from build123d import *

# Parameters (mm, degrees)
F0_W     = 73.131912
F0_H     = 3.448933
F1_DEPTH = 19.05


with BuildPart() as f1:
    # F0 (on Front) → F1 (new body)
    with BuildSketch(Plane.XZ):
        with Locations((-0.653278, -1.724466)):
            Rectangle(F0_W, F0_H)
        Polygon((-37.219234, 0), (-38.690276, 0), (-38.690276, -56.196377), (-37.219234, -56.196377), (-37.219234, -3.448933), align=None)
    extrude(amount=F1_DEPTH)


solid = f1.part
Work out the finished part from the listing and answer in its coordinate system (mm). A direction names the side the tool comes from. Coordinates: 2 decimals unless noted, no trailing zeros. Order: outer loops, then holes, each group sorted by start corner. A loop starts at its lowest first (then second) coordinate and runs counter-clockwise, first axis right, second up. Notation, with made-up numbers: (78.25, 55) - (122.25, 55) arc R19 ccw to (122.25, 84) - close; hole circle Ø5 at (-29.75, 7). An arc over 180 degrees is marked (long way). Put each result on its own line as item: value. Start each with the question number.
1) Find the intervals of material crossed by line 1 (Z direction, x = 23, y = -13.75); line 2 (X direction, y = -12, z = -33), in increasing order. Write a range as from..to.
2) Find section C-C (x = -31). Give the vertices of the cut face in (y, z).
3) Flat-ended cylindrical pins translate along their axes: pin 1 (1 mm diameter, centred on x = 24.5, y = -14, fed in from -Z); pin 2 (1.5 mm diameter, centred on y = -5.5, z = -40.5, fed in from +X). Find the tip coordinate at first contact, or state that the pin passes through.
4) Find section B-B (z = -49.5). Give the vertices of the cut face in (x, y).
5) For faces 1 (the flat face through (-38.69, -9, -28)), 2 (the flat face through (-37.219, -9, -30)), determine the directions among +Z, -Z, +X, -X, +Y, -Y from which every point of the face is accessible in a straight line to the end or side of a thin tool.
6) Find section A-A (y = -11.5). Give the vertices of the cut face in (x, z).
Results list:
1. line 1: z = -3.45..0
1. line 2: x = -38.69..-37.22
2. outline: (-19.05, -3.45) - (0, -3.45) - (0, 0) - (-19.05, 0) - close
3. pin 1: stops at z = -3.45
3. pin 2: stops at x = -37.22
4. outline: (-38.69, -19.05) - (-37.22, -19.05) - (-37.22, 0) - (-38.69, 0) - close
5. face 1: +Z, -Z, -X, +Y, -Y
5. face 2: -Z, +X, +Y, -Y
6. outline: (-38.69, -56.2) - (-37.22, -56.2) - (-37.22, -3.45) - (35.91, -3.45) - (35.91, 0) - (-38.69, 0) - close
